Read the model definition and answer for the solid it produces. Units are mm, in the model's axes. Coordinates: 2 decimals unless noted, no trailing zeros. Loops run counter-clockwise (first coordinate to the right, second up) from the corner with the lowest first, then second, coordinate; pieces in that order, holes last. Notation, with made-up numbers: (89.5, 11.5) -> (148.5, 11.5) arc R24 cw to (148.5, 34.5) -> close; hole circle Ø4 at (41.25, 18.25). An arc over 180 degrees is marked (long way). Answer as a JSON object with one key per item and string values. Group by question number.
Q1. Each of these flat-tipped pins is pushed along its axis until it touches: P1, Ø1, axis at x = -228.5, z = 63.5, coming from the +Y side; P2, Ø2.5, axis at x = -281, y = 5, coming from the -Z side; P3, Ø4, axis at x = -283, y = 3, coming from the +Z side. Where does it stop, or does it pass through?
Q2. The part is cut by section B-B on y = 49. Write down the section's boundary in (x, z), and give its area (3 significant figures).
Q3. The part is cut by section A-A on z = 70.5. Write down the section's boundary in (x, y).
Q4. Straight lines are drawn through the part: line 1 along Y through (x, z) = (-274, 71); line 2 along Y through (x, z) = (-80, 44.5). For each, find the intervals that lie inside material, in ascending order. Write a range as [from, to].
from build123d import *

# Parameters (mm, degrees)
BOSS_EXTRUDE1_DEPTH = 50
SKETCH2_W           = 30
SKETCH2_H           = 2.7
BOSS_EXTRUDE2_DEPTH = 2.7
SKETCH3_W           = 2.743497838
SKETCH3_H           = 100
CUT_EXTRUDE1_DEPTH  = 50
CUT_EXTRUDE2_DEPTH  = 331.140027497


with BuildPart() as part:
    # Sketch1 → Boss-Extrude1 (new body)
    with BuildSketch(Plane.XY):
        Polygon((-300, 0), (-299.146185032, -2.561444905), (0.853814968, 97.438555095), (0, 100), align=None)
    boss_extrude1 = extrude(amount=BOSS_EXTRUDE1_DEPTH)

    # Sketch2 → Boss-Extrude2 (add)
    with BuildSketch(Plane(origin=(-30, 90, 0), x_dir=(0.9486832980505159, 0.3162277660168317, 0), z_dir=(-0.3162277660168318, 0.948683298050516, 0))):
        with Locations((-3.377223398, 1.35)):
            Rectangle(SKETCH2_W, SKETCH2_H)
        with Locations((-123.377223398, 1.35)):
            Rectangle(SKETCH2_W, SKETCH2_H)
        with Locations((-243.377223398, 1.35)):
            Rectangle(SKETCH2_W, SKETCH2_H)
    boss_extrude2 = extrude(amount=-BOSS_EXTRUDE2_DEPTH)

    # Mirror1: Boss-Extrude1 across plane
    add(boss_extrude1.mirror(Plane.XY.offset(50)))

    # Mirror2: Boss-Extrude2 across plane
    add(boss_extrude2.mirror(Plane.XY.offset(50)))

    # Sketch3 → Cut-Extrude1 (cut)
    with BuildSketch(Plane(origin=(-30, 90, 0), x_dir=(0.9486832980505159, 0.3162277660168317, 0), z_dir=(-0.3162277660168318, 0.948683298050516, 0))):
        with Locations((-283.233240496, -50)):
            Rectangle(SKETCH3_W, SKETCH3_H)
    extrude(amount=-CUT_EXTRUDE1_DEPTH, mode=Mode.SUBTRACT)

    # Sketch4 → Cut-Extrude2 (cut, through all)
    with BuildSketch(Plane(origin=(0, 0, 0), x_dir=(-1, 0, 0), z_dir=(0, 0, -1))):
        Polygon((296.543474454, -1.693874712), (297.108099358, 0), (297.397289422, 0.867570193), (292.315665286, 2.561444905), (291.461850318, 0), align=None)
    extrude(amount=-CUT_EXTRUDE2_DEPTH, mode=Mode.SUBTRACT)


solid = part.part
Final values:
{
 "1": {"P1": "stops at y = 24", "P2": "stops at z = 0", "P3": "stops at z = 100"},
 "2": {"outline": "(-153, -2.7) -> (-144.46, -2.7) -> (-144.46, 102.7) -> (-153, 102.7) -> close", "area": "900 mm2"},
 "3": {"outline": "(-292.32, 2.56) -> (-291.46, 0) -> (0.85, 97.44) -> (0, 100) -> close"},
 "4": {"line 1": "y = [5.82, 8.67]", "line 2": "y = [70.49, 73.33]"}
}
